```python
from build123d import *

# Parameters (mm, degrees)
SKETCH_1_W                  = 54
SKETCH_1_H                  = 39
EXTRUDE_1_DEPTH             = 20
SKETCH_2_W                  = 6.5
SKETCH_2_H                  = 28
CUT_EXTRUDE_1_DEPTH         = 42.003048667
SKETCH_3_W                  = 6.5
SKETCH_3_H                  = 28
CUT_EXTRUDE_2_DEPTH         = 42.003048667
SKETCH_4_W                  = 6.5
SKETCH_4_H                  = 8.5
CUT_EXTRUDE_3_DEPTH         = 42.003048667
SKETCH_5_W                  = 5
SKETCH_5_H                  = 2
CUT_EXTRUDE_4_DEPTH         = 42.003048667
CUT_EXTRUDE_5_DEPTH         = 2
SKETCH_7_W                  = 6.5
SKETCH_7_H                  = 6.5
CUT_EXTRUDE_6_DEPTH         = 42.003048667
HOLE_WIZARD_4_2_4_2_1_D     = 4.2
HOLE_WIZARD_4_2_4_2_1_DEPTH = 30.5


with BuildPart() as part:
    # 草图1 → 凸台-拉伸1 (new body)
    with BuildSketch(Plane.XZ.offset(50)):
        with Locations((0, 4)):
            Rectangle(SKETCH_1_W, SKETCH_1_H)
    extrude(amount=-EXTRUDE_1_DEPTH)

    # 草图2 → 切除-拉伸1 (cut, through all)
    with BuildSketch(Plane(origin=(0, -30, 0), x_dir=(-1, 0, 0), z_dir=(0, 1, 0))):
        with Locations((-23.75, 9.5)):
            Rectangle(SKETCH_2_W, SKETCH_2_H)
    extrude(amount=-CUT_EXTRUDE_1_DEPTH, mode=Mode.SUBTRACT)

    # 草图3 → 切除-拉伸2 (cut, through all)
    with BuildSketch(Plane(origin=(0, -30, 0), x_dir=(-1, 0, 0), z_dir=(0, 1, 0))):
        with Locations((23.75, 9.5)):
            Rectangle(SKETCH_3_W, SKETCH_3_H)
    extrude(amount=-CUT_EXTRUDE_2_DEPTH, mode=Mode.SUBTRACT)

    # 草图4 → 切除-拉伸3 (cut, through all)
    with BuildSketch(Plane(origin=(0, -30, 0), x_dir=(-1, 0, 0), z_dir=(0, 1, 0))):
        with Locations((23.75, -11.25)):
            Rectangle(SKETCH_4_W, SKETCH_4_H)
    extrude(amount=-CUT_EXTRUDE_3_DEPTH, mode=Mode.SUBTRACT)

    # 草图5 → 切除-拉伸4 (cut, through all)
    with BuildSketch(Plane(origin=(0, -30, 0), x_dir=(-1, 0, 0), z_dir=(0, 1, 0))):
        with Locations((18, -14.5)):
            Rectangle(SKETCH_5_W, SKETCH_5_H)
    extrude(amount=-CUT_EXTRUDE_4_DEPTH, mode=Mode.SUBTRACT)

    # 草图6 → 切除-拉伸5 (cut)
    with BuildSketch(Plane(origin=(0, 0, -15.5), x_dir=(-1, 0, 0), z_dir=(0, 0, -1))):
        with BuildLine():
            Line((-10.5, -30), (-27, -30))
            Line((-27, -30), (-27, -50))
            Line((-27, -50), (-10.5, -50))
            ThreePointArc((-10.5, -50), (-20.5, -40), (-10.5, -30))
        make_face()
    extrude(amount=-CUT_EXTRUDE_5_DEPTH, mode=Mode.SUBTRACT)

    # 草图7 → 切除-拉伸6 (cut, through all)
    with BuildSketch(Plane(origin=(0, -30, 0), x_dir=(-1, 0, 0), z_dir=(0, 1, 0))):
        with Locations((-23.75, -10.25)):
            Rectangle(SKETCH_7_W, SKETCH_7_H)
    extrude(amount=-CUT_EXTRUDE_6_DEPTH, mode=Mode.SUBTRACT)

    # 草图8 → 旋转1 (revolve)
    with BuildSketch(Plane(origin=(0, -40, 0), x_dir=(1, 0, 0), z_dir=(0, 1, 0))):
        Polygon((13.5, 22), (10.5, 22), (10.5, 15.5), (17, 15.5), (17, 17), (13.5, 17), align=None)
    revolve(axis=Axis((10.5, -40, -22), (0, 0, 1)))

    # Ø4.2 (4.2) 直径孔1
    with Locations(Plane(origin=(0, 0, -7), x_dir=(-1, 0, 0), z_dir=(0, 0, -1))):
        with Locations((24.1, -45), (24.1, -35), (-24.1, -45), (-24.1, -35)):
            Hole(HOLE_WIZARD_4_2_4_2_1_D / 2, depth=HOLE_WIZARD_4_2_4_2_1_DEPTH)


solid = part.part
```
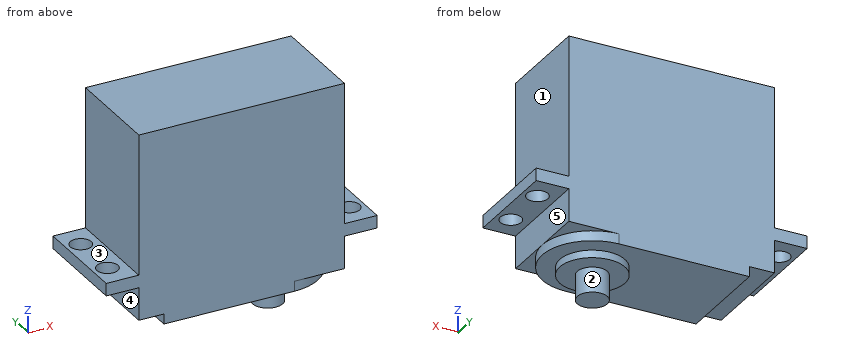
Part model, mm, in its own coordinate system. Face numbers are marked on the shaded views. A direction names the side the tool comes from. Coordinates: 2 decimals unless noted, no trailing zeros. Loops run counter-clockwise (first coordinate to the right, second up) from the corner with the lowest first, then second, coordinate; pieces in that order, holes last. Notation, with made-up numbers: (-22, -25.75) - (0, -25.75) arc R29 ccw to (0, -3.75) - close; hole circle Ø5 at (-5.75, 42.25). An arc over 180 degrees is marked (long way). Write item = value, one per line. Start each with the question number.
Item 1: Cut at C-C, the plane y = -45. Give the cut face in (x, z), and give its area (3 significant figures).
Item 2: Wall check: L1, parallel to Y at x = -24.1, z = -5.65; L2, parallel to Z at x = 15, y = -41.25; L3, parallel to X at y = -45.75, z = -12.5. Give the ranges that are in metal, low to high. Write a range as from..to.
Item 3: Cut at B-B, the plane x = 24.1. Give the cut face in (y, z).
Item 4: Flat gauge pins, fed straight in: pin 1 Ø2.5 at (x, y) = (-24.1, -45) entering from -Z; pin 2 Ø6 at (y, z) = (-35, 6.5) entering from -X; pin 3 Ø6 at (x, y) = (-3.5, -41.5) entering from -Z; pin 4 Ø11 at (x, y) = (14, -36) entering from -Z. Where does each tip first touch, or does it go through?
Item 5: Cut at D-D, the plane y = -47.75. Give the cut face in (x, z).
Item 6: Cut at A-A, the plane z = -6. Give the cut face in (x, y).
Item 7: 3-axis set-ups, long thin cutter, end or side, ignore diameter. For the marked faces 1, 2, 3, 4 and 5: which of +Z, -Z, +X, -X, +Y, -Y reach the whole face in a straight line?
The answers:
q1.outline = (-27, -7) - (-26.2, -7) - (-26.2, -4.5) - (-27, -4.5) - close; (-22, -7) - (-20.5, -7) - (-20.5, -13.5) - (-15.5, -13.5) - (-15.5, -15.5) - (6.35, -15.5) - (6.35, -17) - (14.65, -17) - (14.65, -15.5) - (19.16, -15.5) - (19.16, -13.5) - (20.5, -13.5) - (20.5, -7) - (22, -7) - (22, -4.5) - (20.5, -4.5) - (20.5, 23.5) - (-20.5, 23.5) - (-20.5, -4.5) - (-22, -4.5) - close; (26.2, -7) - (27, -7) - (27, -4.5) - (26.2, -4.5) - close
q1.area = 1,610 mm2
q2.L1 = -50..-47.1, -42.9..-37.1, -32.9..-30
q2.L2 = -17..23.5
q2.L3 = -20.5..20.5
q3.outline = (-50, -7) - (-47.1, -7) - (-47.1, -4.5) - (-50, -4.5) - close; (-42.9, -7) - (-37.1, -7) - (-37.1, -4.5) - (-42.9, -4.5) - close; (-32.9, -7) - (-30, -7) - (-30, -4.5) - (-32.9, -4.5) - close
q4.pin_1 = through
q4.pin_2 = -20.5
q4.pin_3 = -15.5
q4.pin_4 = -22
q5.outline = (-27, -7) - (-20.5, -7) - (-20.5, -13.5) - (-15.5, -13.5) - (-15.5, -15.5) - (16.82, -15.5) - (16.82, -13.5) - (20.5, -13.5) - (20.5, -7) - (27, -7) - (27, -4.5) - (20.5, -4.5) - (20.5, 23.5) - (-20.5, 23.5) - (-20.5, -4.5) - (-27, -4.5) - close
q6.outline = (-27, -50) - (27, -50) - (27, -30) - (-27, -30) - close; hole circle Ø4.2 at (-24.1, -45); hole circle Ø4.2 at (-24.1, -35); hole circle Ø4.2 at (24.1, -45); hole circle Ø4.2 at (24.1, -35)
q7.face_1 = +Z, +X, +Y, -Y
q7.face_2 = -Z
q7.face_3 = +Z, -X, +Y, -Y
q7.face_4 = -Z, -X, +Y, -Y
q7.face_5 = -Z, +X, +Y, -Y
